Could you check a few things on this model? Use its own coordinates, in mm. Give positions to 0.01 mm unless a question says otherwise; leave off trailing zeros. Loops run counter-clockwise (first coordinate to the right, second up) from the corner with the lowest first, then second, coordinate; pieces in that order, holes last. Notation, with made-up numbers: (-13.75, 66) - (15.25, 66) arc R34 cw to (15.25, 96) - close; hole circle Ø7 at (-37.5, -2.5). An arc over 180 degrees is marked (long way). Use CSV: the item, a comma, the result in double quotes.
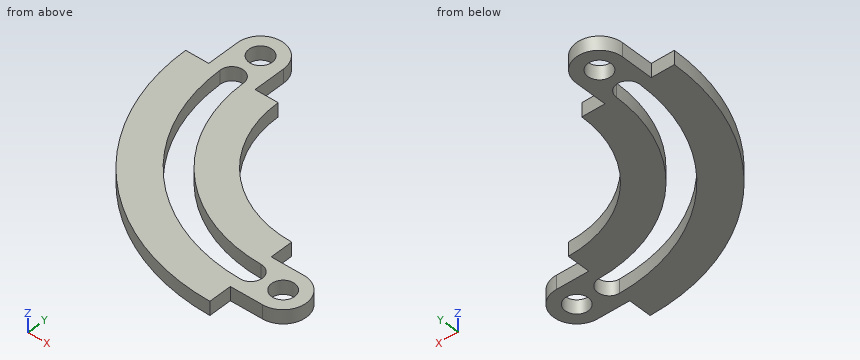
from build123d import *

# Parameters (mm, degrees)
SALIENTE_EXTRUIR1_DEPTH = 6
CROQUIS3_R              = 5
CORTAR_EXTRUIR1_DEPTH   = 6
CORTAR_EXTRUIR3_DEPTH   = 6


with BuildPart() as part:
    # cuadrado → Saliente-Extruir1 (new body)
    with BuildSketch(Plane.XY):
        with BuildLine():
            Line((-50, 90), (-60, 90))
            Line((-60, 90), (-60, 104))
            ThreePointArc((-60, 104), (-70, 114), (-80, 104))
            Line((-80, 104), (-80, 90))
            Line((-80, 90), (-90, 90))
            ThreePointArc((-90, 90), (-63.639610307, 26.360389693), (0, 0))
            Line((0, 0), (0, 10))
            Line((0, 10), (14, 10))
            ThreePointArc((14, 10), (24, 20), (14, 30))
            Line((14, 30), (0, 30))
            Line((0, 30), (0, 40))
            ThreePointArc((0, 40), (-35.355339059, 54.644660941), (-50, 90))
        make_face()
    extrude(amount=SALIENTE_EXTRUIR1_DEPTH)

    # Croquis3 → Cortar-Extruir1 (cut)
    with BuildSketch(Plane.XY):
        with Locations((-70, 104)):
            Circle(CROQUIS3_R)
        with Locations((14, 20)):
            Circle(CROQUIS3_R)
    extrude(amount=CORTAR_EXTRUIR1_DEPTH, mode=Mode.SUBTRACT)

    # Croquis4 → Cortar-Extruir3 (cut)
    with BuildSketch(Plane.XY):
        with BuildLine():
            ThreePointArc((-74.999538142, 89.951945487), (-52.836185081, 37.163814919), (-0.048054513, 15.000461858))
            ThreePointArc((-0.048054513, 15.000461858), (4.999769071, 19.952176416), (0.048054513, 25))
            ThreePointArc((0.048054513, 25), (-45.765117269, 44.234882731), (-65, 90.048054513))
            ThreePointArc((-65, 90.048054513), (-70.047823584, 94.999769071), (-74.999538142, 89.951945487))
        make_face()
    extrude(amount=CORTAR_EXTRUIR3_DEPTH, mode=Mode.SUBTRACT)


solid = part.part
1) Suppose I cut it at A-A (y = 49). Please give me the cut outline in (x, z).
Answer below:
outline,"(-80.12, 0) - (-62.49, 0) - (-62.49, 6) - (-80.12, 6) - close; (-50.08, 0) - (-28.62, 0) - (-28.62, 6) - (-50.08, 6) - close"
2) Suppose I cut it at B-B (x = 2.5). Please give me the cut outline in (y, z).
Answer below:
outline,"(10, 0) - (15.67, 0) - (15.67, 6) - (10, 6) - close; (24.33, 0) - (30, 0) - (30, 6) - (24.33, 6) - close"
3) Suppose I cut it at C-C (x = -72.5). Please give me the cut outline in (y, z), plus the area to 3 significant figures.
Answer below:
outline,"(36.67, 0) - (71.38, 0) - (71.38, 6) - (36.67, 6) - close; (94.33, 0) - (99.67, 0) - (99.67, 6) - (94.33, 6) - close; (108.33, 0) - (113.68, 0) - (113.68, 6) - (108.33, 6) - close"
area,"272 mm2"
4) I need wall thicknesses on line 1 along X through (y, z) = (22.5, 0.75); line 2 along Y through (x, z) = (14, 2.35); line 3 along X through (y, z) = (21.5, 3.5). Which ranges of each line are inside material? Lowest first, please.
Answer below:
line 1,"x = -59.53 to -32.17, 4.33 to 9.67, 18.33 to 23.68"
line 2,"y = 10 to 15, 25 to 30"
line 3,"x = -58.38 to -30.01, 4.77 to 9.23, 18.77 to 23.89"
5) I'm going to push flat-ended pins straight in: P1, Ø2, axis at x = -43, z = 2.5, coming from the +Y side; P2, Ø3, axis at y = 96.5, z = 2.5, coming from the +X side; P3, Ø1.8, axis at y = 96, z = 2.5, coming from the -X side. Where does each tip first touch, or does it pass through?
Answer below:
P1,"stops at y = 66.25"
P2,"stops at x = -60"
P3,"stops at x = -80"
6) Suppose I cut it at D-D (y = 20). Please give me the cut outline in (x, z), plus the area to 3 significant figures.
Answer below:
outline,"(-56.57, 0) - (-26.38, 0) - (-26.38, 6) - (-56.57, 6) - close; (5, 0) - (9, 0) - (9, 6) - (5, 6) - close; (19, 0) - (24, 0) - (24, 6) - (19, 6) - close"
area,"235 mm2"
